from build123d import *

# Parameters (mm, degrees)
F1_DEPTH = 10
F2_W     = 7.5
F2_H     = 10
F3_DEPTH = 1.5
F4_W     = 7.5
F4_H     = 10
F5_DEPTH = 1.5


with BuildPart() as f1:
    # F0 (on Top) → F1 (new body)
    with BuildSketch(Plane.XY):
        Polygon((58, 0), (0, 0), (0, -15), (73, -15), (73, 10), (58, 10), align=None)
    extrude(amount=F1_DEPTH)

    # F2 (on face) → F3 (cut)
    with BuildSketch(Plane(origin=(0, 0, 0), x_dir=(0, -1, 0), z_dir=(-1, 0, 0))):
        with Locations((3.75, 5)):
            Rectangle(F2_W, F2_H)
    extrude(amount=-F3_DEPTH, mode=Mode.SUBTRACT)

    # F4 (on face) → F5 (join)
    with BuildSketch(Plane(origin=(0, 0, 0), x_dir=(0, -1, 0), z_dir=(-1, 0, 0))):
        with Locations((11.25, 5)):
            Rectangle(F4_W, F4_H)
    extrude(amount=F5_DEPTH)


solid = f1.part
Check sheet for the modelled part. Datum: model origin and axes. Units: mm. A direction names the side the tool comes from. Give positions to 0.01 mm unless a question says otherwise; leave off trailing zeros. Write each loop counter-clockwise with the first axis right and the second up, starting at its lowest first coordinate (ties: lowest second). Pieces come first, ordered by that corner, then holes. Notation, with made-up numbers: (56, 18) -> (73, 18) arc R18 ccw to (73, 31) -> close; hole circle Ø5 at (84.25, 87). An arc over 180 degrees is marked (long way). One line per item, written item: value. Start each with the question number.
Item 1: Section check A-A on z = 6.5. Record the cut outline in (x, y), then the cut area to 4 significant figures.
Item 2: Tool access check on faces 1 (the flat face through (0, -7.5, 5)), 2 (the flat face through (45, -5, 10)). Record the directions out of +Z, -Z, +X, -X, +Y, -Y that give a thin tool (end or side, any length) a straight path to the whole face; none if there is none.
Item 3: Gauge pin test, flat ends, axial feed: pin 1 (2.5 mm diameter, centred on x = 0, z = 3.5, fed in from +Y); pin 2 (1.5 mm diameter, centred on y = 1.5, z = 6, fed in from -X); pin 3 (5 mm diameter, centred on x = 33, z = 5, fed in from +Y). Record the tip position at first contact, or that the pin passes through.
Item 4: Section check C-C on x = 51. Record the cut outline in (y, z).
Item 5: Section check B-B on y = -4. Record the cut outline in (x, z), then the cut area to 3 significant figures.
Item 6: Material ranges on probe 1 along X at (y, z) = (-5.5, 0.5); probe 2 along Y at (x, z) = (36.5, 9.25); probe 3 along X at (y, z) = (4.5, 2.5), recorded low to high. Write a range as from..to.
Results list:
1. outline: (-1.5, -15) -> (73, -15) -> (73, 10) -> (58, 10) -> (58, 0) -> (1.5, 0) -> (1.5, -7.5) -> (-1.5, -7.5) -> close
1. area: 1,245 mm²
2. face 1: +Z, -Z, -X, +Y
2. face 2: +Z, +X, -X, +Y, -Y
3. pin 1: y = -7.5
3. pin 2: x = 58
3. pin 3: y = 0
4. outline: (-15, 0) -> (0, 0) -> (0, 10) -> (-15, 10) -> close
5. outline: (1.5, 0) -> (73, 0) -> (73, 10) -> (1.5, 10) -> close
5. area: 715 mm²
6. probe 1: 1.5..73
6. probe 2: -15..0
6. probe 3: 58..73
